from build123d import *

# Parameters (mm, degrees)
BOSS_EXTRUDE1_DEPTH = 20
SKETCH2_R           = 5
CUT_EXTRUDE1_DEPTH  = 67.580778007
SKETCH3_R           = 2.5
CUT_EXTRUDE2_DEPTH  = 65.226162893
SKETCH4_R           = 1.5
BOSS_EXTRUDE2_DEPTH = 7


with BuildPart() as part:
    # Sketch1 → Boss-Extrude1 (new, symmetric)
    with BuildSketch(Plane.XY):
        Polygon((0, 0), (0, 35), (7, 35), (7, 7), (57, 7), (57, 0), align=None)
    extrude(amount=BOSS_EXTRUDE1_DEPTH, both=True)

    # Sketch2 → Cut-Extrude1 (cut, through all)
    with BuildSketch(Plane(origin=(0, 7, 0), x_dir=(1, 0, 0), z_dir=(0, 1, 0))):
        with Locations(Location((40, 0, 0), (0, 0, 270))):
            Circle(SKETCH2_R)
    extrude(amount=-CUT_EXTRUDE1_DEPTH, mode=Mode.SUBTRACT)

    # Sketch3 → Cut-Extrude2 (cut, through all)
    with BuildSketch(Plane(origin=(7, 0, 0), x_dir=(0, 0, -1), z_dir=(1, 0, 0))):
        with Locations(Location((12, 27, 0), (0, 0, 90))):
            Circle(SKETCH3_R)
        with Locations(Location((12, 15, 0), (0, 0, 90))):
            Circle(SKETCH3_R)
        with Locations(Location((-12, 27, 0), (0, 0, 90))):
            Circle(SKETCH3_R)
        with Locations(Location((-12, 15, 0), (0, 0, 90))):
            Circle(SKETCH3_R)
    extrude(amount=-CUT_EXTRUDE2_DEPTH, mode=Mode.SUBTRACT)

    # Sketch4 → Boss-Extrude2 (add)
    # profile 1 of 2: a face of its own
    with BuildSketch(Plane(origin=(0, 7, 0), x_dir=(1, 0, 0), z_dir=(0, 1, 0))):
        with BuildLine():
            Line((36.764961653, 24.852557521), (33.236125371, 20))
            Line((33.236125371, 20), (46.763874629, 20))
            Line((46.763874629, 20), (43.235038347, 24.852557521))
            ThreePointArc((43.235038347, 24.852557521), (40, 26.5), (36.764961653, 24.852557521))
        make_face()
        with Locations(Location((40, 22.5, 0), (0, 0, 270))):
            Circle(SKETCH4_R, mode=Mode.SUBTRACT)
    # profile 2 of 2: a face of its own
    with BuildSketch(Plane(origin=(0, 7, 0), x_dir=(1, 0, 0), z_dir=(0, 1, 0))):
        with BuildLine():
            Line((43.235038347, -24.852557521), (46.763874629, -20))
            Line((46.763874629, -20), (33.236125371, -20))
            Line((33.236125371, -20), (36.764961653, -24.852557521))
            ThreePointArc((36.764961653, -24.852557521), (40, -26.5), (43.235038347, -24.852557521))
        make_face()
        with Locations(Location((40, -22.5, 0), (0, 0, 270))):
            Circle(SKETCH4_R, mode=Mode.SUBTRACT)
    extrude(amount=-BOSS_EXTRUDE2_DEPTH)


solid = part.part
Design review of the part built by this model. Coordinates are the model's own, in mm. A direction names the side the tool comes from. Round coordinates to 2 decimals unless told otherwise and drop trailing zeros. Loops run counter-clockwise (first coordinate to the right, second up) from the corner with the lowest first, then second, coordinate; pieces in that order, holes last. Notation, with made-up numbers: (-25, -14) -> (-1, -14) arc R17 ccw to (-1, 18) -> close; hole circle Ø3 at (76.25, 2.25). An arc over 180 degrees is marked (long way). Use one line per item in the form item = value. Start each with the question number.
Q1. We need section B-B on z = 0. Give the boundary of the cut face in (x, y), then the cut area to 3 significant figures.
Q2. We need section D-D on x = 6. Give the boundary of the cut face in (y, z), then the cut area to 3 significant figures.
Q3. Machinability: for faces 1 (the face through (52, 4, 20)), 2 (the face through (52, 4, -20)), 3 (the face through (32, 7, 0)), which of the approach directions +Z, -Z, +X, -X, +Y, -Y give a long, thin tool a straight path to every point of the face, cutting with its end or side? Answer none if there is none.
Q4. For pin 1 Ø2 at (y, z) = (30, 3) entering from +X; pin 2 Ø5.5 at (x, y) = (54, 4) entering from -Z; pin 3 Ø1 at (x, z) = (20, -11) entering from +Y, all flat-tipped, find the tip position at first contact; note any pin that passes through.
Q5. Wall thickness on line 1 along Z through (x, y) = (3, 27); line 2 along X through (y, z) = (5, 0); line 3 along Y through (x, z) = (53, -3): over which ranges is each line inside the solid? List them lowest first. Write a range as [from, to].
Q6. Draft analysis for pull direction X (two halves, no side actions). For faces 4 (the face through (34.976, 3.549, 22.392)), 5 (the face through (38.536, 3.549, -22.825)), 6 (the face through (45.024, 3.549, -22.392)), 7 (the face through (6, 10, 20)), state which applies: +X half, -X half, draft (parallel to the pull), parting line (faces both ways), or undercut.
Q7. We need section C-C on y = 27. Give the boundary of the cut face in (x, z).
Q8. We need section A-A on x = 40. Give the boundary of the cut face in (y, z), then the cut area to 3 significant figures.
Calculated:
q1.outline = (0, 0) -> (35, 0) -> (35, 7) -> (7, 7) -> (7, 35) -> (0, 35) -> close; (45, 0) -> (57, 0) -> (57, 7) -> (45, 7) -> close
q1.area = 525 mm²
q2.outline = (0, -20) -> (35, -20) -> (35, 20) -> (0, 20) -> close; hole circle Ø5 at (15, -12); hole circle Ø5 at (15, 12); hole circle Ø5 at (27, -12); hole circle Ø5 at (27, 12)
q2.area = 1,320 mm²
q3.face_1 = +Z, +X, +Y, -Y
q3.face_2 = -Z, +X, +Y, -Y
q3.face_3 = +Z, -Z, +X, +Y
q4.pin_1 = 7
q4.pin_2 = -20
q4.pin_3 = 7
q5.line_1 = [-20, -14.5], [-9.5, 9.5], [14.5, 20]
q5.line_2 = [0, 35], [45, 57]
q5.line_3 = [0, 7]
q6.face_4 = -X half
q6.face_5 = undercut
q6.face_6 = +X half
q6.face_7 = draft
q7.outline = (0, -20) -> (7, -20) -> (7, -14.5) -> (0, -14.5) -> close; (0, -9.5) -> (7, -9.5) -> (7, 9.5) -> (0, 9.5) -> close; (0, 14.5) -> (7, 14.5) -> (7, 20) -> (0, 20) -> close
q8.outline = (0, -26.5) -> (7, -26.5) -> (7, -24) -> (0, -24) -> close; (0, -21) -> (7, -21) -> (7, -5) -> (0, -5) -> close; (0, 5) -> (7, 5) -> (7, 21) -> (0, 21) -> close; (0, 24) -> (7, 24) -> (7, 26.5) -> (0, 26.5) -> close
q8.area = 259 mm²
